from build123d import *

# Parameters (mm, degrees)
SKETCH1_R             = 25
BOSS_EXTRUDE1_DEPTH   = 2
SKETCH2_R             = 1.5
CUT_EXTRUDE1_DEPTH    = 3
BOSS_EXTRUDE2_DEPTH   = 7
CUT_EXTRUDE2_DEPTH    = 7
M4_TAPPED_HOLE1_D     = 3.3
M4_TAPPED_HOLE1_DEPTH = 5
M4_TAPPED_HOLE2_D     = 3.3


with BuildPart() as part:
    # Sketch1 → Boss-Extrude1 (new body)
    with BuildSketch(Plane(origin=(0, 0, 0), x_dir=(1, 0, 0), z_dir=(0, 1, 0))):
        with Locations(Location((0, 0, 0), (0, 0, 270))):
            Circle(SKETCH1_R)
    extrude(amount=BOSS_EXTRUDE1_DEPTH)

    # Sketch2 → Cut-Extrude1 (cut)
    with BuildSketch(Plane(origin=(0, 2, 0), x_dir=(1, 0, 0), z_dir=(0, 1, 0))):
        with Locations(Location((0, 20, 0), (0, 0, 270))):
            Circle(SKETCH2_R)
        with Locations(Location((20, 0, 0), (0, 0, 270))):
            Circle(SKETCH2_R)
        with Locations(Location((0, -20, 0), (0, 0, 270))):
            Circle(SKETCH2_R)
        with Locations(Location((-20, 0, 0), (0, 0, 270))):
            Circle(SKETCH2_R)
    extrude(amount=-CUT_EXTRUDE1_DEPTH, mode=Mode.SUBTRACT)

    # Sketch3 → Boss-Extrude2 (add)
    with BuildSketch(Plane(origin=(0, 2, 0), x_dir=(1, 0, 0), z_dir=(0, 1, 0))):
        Polygon((0, 11.547005384), (-10, 5.773502692), (-10, -5.773502692), (0, -11.547005384), (10, -5.773502692), (10, 5.773502692), align=None)
    extrude(amount=BOSS_EXTRUDE2_DEPTH)

    # Sketch4 → Cut-Extrude2 (cut)
    with BuildSketch(Plane.XZ):
        Polygon((0, 5.773502692), (-5, 2.886751346), (-5, -2.886751346), (0, -5.773502692), (5, -2.886751346), (5, 2.886751346), align=None)
    extrude(amount=-CUT_EXTRUDE2_DEPTH, mode=Mode.SUBTRACT)

    # M4 Tapped Hole1
    with Locations(Plane.ZY.offset(10)):
        with Locations((0, 5)):
            Hole(M4_TAPPED_HOLE1_D / 2, depth=M4_TAPPED_HOLE1_DEPTH)

    # M4 Tapped Hole2 (through all)
    with Locations(Plane(origin=(0, 9, 0), x_dir=(1, 0, 0), z_dir=(0, 1, 0))):
        with Locations((0, 0)):
            Hole(M4_TAPPED_HOLE2_D / 2)


solid = part.part
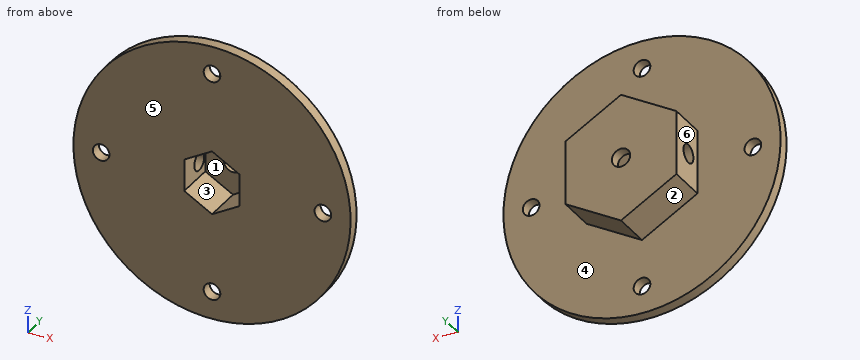
Can you work these out from the model? Positions are in its coordinate system, mm. Face numbers are marked on the shaded views. A direction names the side the tool comes from. Coordinates: 2 decimals unless noted, no trailing zeros. Loops run counter-clockwise (first coordinate to the right, second up) from the corner with the lowest first, then second, coordinate; pieces in that order, holes last. Notation, with made-up numbers: (26, 78.25) - (40, 78.25) arc R27 ccw to (40, 107.25) - close; hole circle Ø6 at (52, -15). An arc over 180 degrees is marked (long way). Put each result on its own line as item: value. Start each with the question number.
Item 1: Suppose I cut it at B-B (z = -20). Please give me the cut outline in (x, y), and give its area (3 significant figures).
Item 2: Suppose I cut it at C-C (x = -20). Please give me the cut outline in (y, z).
Item 3: Which directions (+Z, -Z, +X, -X, +Y, -Y) give clear straight access to the entire face, cutting with the end or side of a thin tool? Please do the marked faces 5 and 6.
Item 4: Suppose I cut it at D-D (z = 0). Please give me the cut outline in (x, y), and give its area (3 significant figures).
Item 5: For pin 1 (4.5 mm diameter, centred on x = 0, z = 0, fed in from +Y); pin 2 (2 mm diameter, centred on x = -5, y = 1.5, fed in from -Z); pin 3 (2 mm diameter, centred on y = 5.5, z = 0, fed in from +X); pin 4 (2 mm diameter, centred on x = -2.5, y = 1.5, fed in from -Z), each with a flat end and sliding along its axis, tell me the tip position at first contact or that it passes through.
Item 6: If I drill on line 1 along X through (y, z) = (0.65, 0); line 2 along Z through (x, y) = (0, 7.75); line 3 along Y through (x, z) = (-7, 0), over which ranges is the centre line in solid material (lowest first)?
Item 7: If we mould it in two halves opening along Z, with no side actions, what happens to the marked faces 1, 2, 3 and 4? For each: +Z half, -Z half, draft (parallel to the pull), parting line (faces both ways), or undercut.
Item 8: Suppose I cut it at A-A (y = 1). Please give me the cut outline in (x, z).
Here are the results:
1. outline: (-15, 0) - (-1.5, 0) - (-1.5, 2) - (-15, 2) - close; (1.5, 0) - (15, 0) - (15, 2) - (1.5, 2) - close
1. area: 54.0 mm²
2. outline: (0, -15) - (2, -15) - (2, -1.5) - (0, -1.5) - close; (0, 1.5) - (2, 1.5) - (2, 15) - (0, 15) - close
3. face 5: +Z, -Z, +X, -X, -Y
3. face 6: +Z, -Z, -X, +Y
4. outline: (-25, 0) - (-21.5, 0) - (-21.5, 2) - (-25, 2) - close; (-18.5, 0) - (-5, 0) - (-5, 3.35) - (-10, 3.35) - (-10, 2) - (-18.5, 2) - close; (-10, 6.65) - (-5, 6.65) - (-5, 7) - (-1.65, 7) - (-1.65, 9) - (-10, 9) - close; (1.65, 7) - (5, 7) - (5, 0) - (18.5, 0) - (18.5, 2) - (10, 2) - (10, 9) - (1.65, 9) - close; (21.5, 0) - (25, 0) - (25, 2) - (21.5, 2) - close
4. area: 135 mm²
5. pin 1: y = 9
5. pin 2: z = -24.68
5. pin 3: x = 10
5. pin 4: z = -24.95
6. line 1: -25 to -21.5, -18.5 to -5, 5 to 18.5, 21.5 to 25
6. line 2: -11.55 to -1.65, 1.65 to 11.55
6. line 3: 0 to 3.35, 6.65 to 9
7. face 1: undercut
7. face 2: -Z half
7. face 3: undercut
7. face 4: draft
8. outline: circle Ø50 at (0, 0); hole circle Ø3 at (-20, 0); hole (-5, -2.89) - (0, -5.77) - (5, -2.89) - (5, 2.89) - (0, 5.77) - (-5, 2.89) - close; hole circle Ø3 at (0, -20); hole circle Ø3 at (0, 20); hole circle Ø3 at (20, 0)
